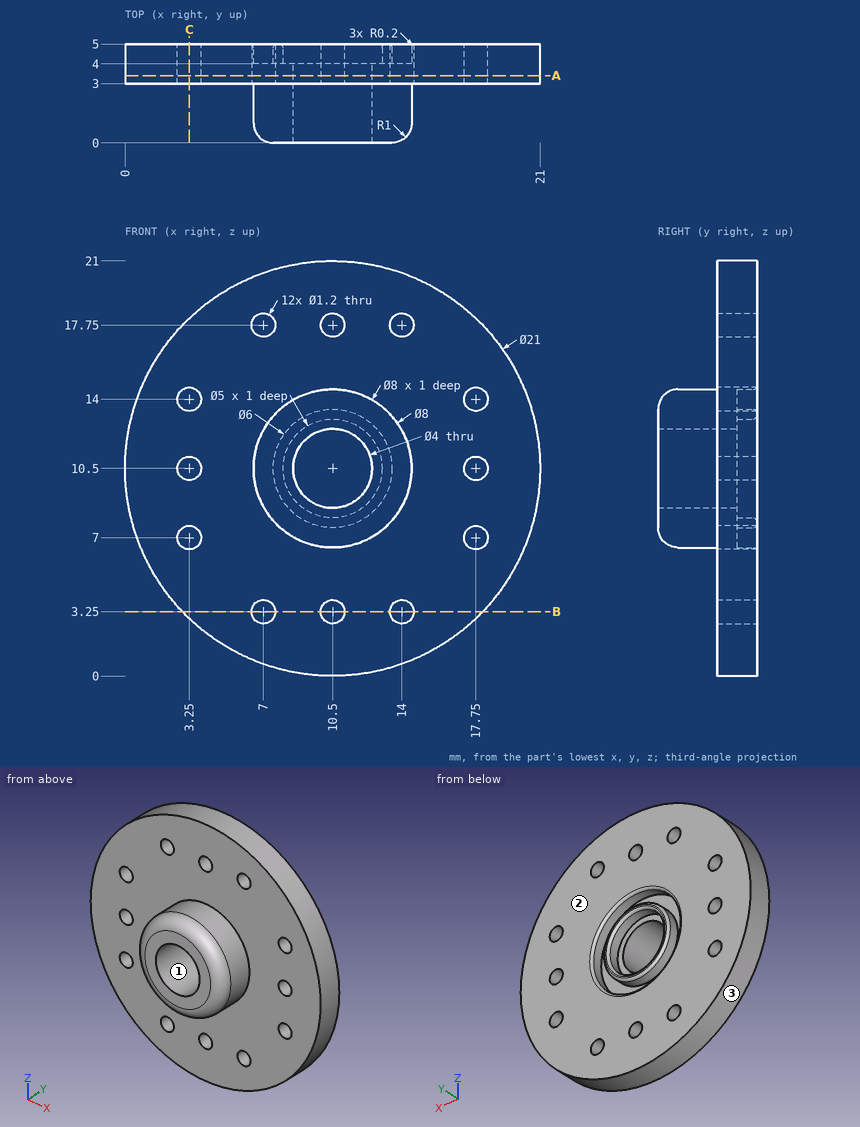
Drawing for the job (mm, zero at the part's lowest x, y, z). Give positions to 0.01 mm unless a question says otherwise; leave off trailing zeros. Order: outer loops, then holes, each group sorted by start corner. A loop starts at its lowest first (then second) coordinate and runs counter-clockwise, first axis right, second up. Notation, with made-up numbers: M 85,-24 L 140,-24 A35 cw 140,14 Z; hole C -32.5,12.25 d5. An arc over 180 degrees is marked long. Use a Markdown table: item, result. Add a question column.
(1) Saw through at A-A, the plane y = 3.4. Give the number of separate pieces and of enclosed holes in the cut face, and give its area (3 significant figures).
(2) Drop flat-ended pins along their axis: P1, Ø1, axis at y = 1, z = 5, coming from the +X side; P2, Ø1.9, axis at x = 7, z = 3.25, coming from the -Y side. Give the stop position or say it passes through.
(3) Saw through at B-B, the plane z = 3.25. Give the cut face in (x, y).
(4) Mould opens along Z. For the marked faces 1, 2 and 3 say: +Z half, -Z half, draft (parallel to the pull), parting line (faces both ways), or undercut.
(5) Probe line 1 along X through (y, z) = (4.65, 10.5); line 2 along Z through (x, y) = (10.5, 3.35); line 3 along X through (y, z) = (3.1, 3.5). List the from-to ranges inside material, lowest first. Write a range as [from, to].
(6) Saw through at C-C, the plane x = 3.25. Give the cut face in (y, z), and give its area (3 significant figures).
Answer key:
| question | item | result |
|---|---|---|
| 1 | separate pieces | 1 |
| 1 | enclosed holes | 13 |
| 1 | area | 320 mm^2 |
| 2 | P1 | through |
| 2 | P2 | y = 3 |
| 3 | outline | M 2.9,3 L 6.4,3 L 6.4,5 L 2.9,5 Z; M 7.6,3 L 9.9,3 L 9.9,5 L 7.6,5 Z; M 11.1,3 L 13.4,3 L 13.4,5 L 11.1,5 Z; M 14.6,3 L 18.1,3 L 18.1,5 L 14.6,5 Z |
| 4 | face 1 | undercut |
| 4 | face 2 | draft |
| 4 | face 3 | parting line |
| 5 | line 1 | [0, 2.65], [3.85, 6.5], [7.5, 8], [13, 13.5], [14.5, 17.15], [18.35, 21] |
| 5 | line 2 | [0, 2.65], [3.85, 8.5], [12.5, 17.15], [18.35, 21] |
| 5 | line 3 | [2.67, 6.45], [7.55, 9.95], [11.05, 13.45], [14.55, 18.33] |
| 6 | outline | M 3,2.9 L 5,2.9 L 5,6.4 L 3,6.4 Z; M 3,7.6 L 5,7.6 L 5,9.9 L 3,9.9 Z; M 3,11.1 L 5,11.1 L 5,13.4 L 3,13.4 Z; M 3,14.6 L 5,14.6 L 5,18.1 L 3,18.1 Z |
| 6 | area | 23.2 mm^2 |
